from build123d import *

# Parameters (mm, degrees)
SKETCH1_W           = 12.1
SKETCH1_H           = 22.8
BOSS_EXTRUDE1_DEPTH = 24.85
SKETCH2_OUTSIDE_W   = 31.966
SKETCH2_OUTSIDE_H   = 34.016
CUT_EXTRUDE1_DEPTH  = 24.85
SKETCH3_R           = 2.875
SKETCH3_R_2         = 6.05
BOSS_EXTRUDE2_DEPTH = 4.65
BOSS_EXTRUDE3_START = 20.8
BOSS_EXTRUDE3_DEPTH = 2.12
CUT_EXTRUDE2_START  = -2.5
SKETCH6_W           = 12.1
SKETCH6_H           = 22.8
SKETCH6_W_2         = 11.9
SKETCH6_H_2         = 22.6
CUT_EXTRUDE2_DEPTH  = 14
SKETCH8_R           = 3.625
BOSS_EXTRUDE5_DEPTH = 0.3
FILLET1_R           = 0.2
SKETCH9_R           = 2.375
CUT_EXTRUDE3_DEPTH  = 1


with BuildPart() as part:
    # Sketch1 → Boss-Extrude1 (new body)
    with BuildSketch(Plane(origin=(0, 0, 0), x_dir=(1, 0, 0), z_dir=(0, 1, 0))):
        Rectangle(SKETCH1_W, SKETCH1_H)
    extrude(amount=BOSS_EXTRUDE1_DEPTH)

    # Sketch2 outside → Cut-Extrude1 (cut)
    with BuildSketch(Plane.ZY.offset(6.05)):
        with Locations((0, 12.425)):
            Rectangle(SKETCH2_OUTSIDE_W, SKETCH2_OUTSIDE_H)
        Polygon((-11.4, 23.85), (-4.47179677, 24.85), (11.4, 24.85), (11.4, 0), (-11.4, 0), align=None, mode=Mode.SUBTRACT)
    extrude(amount=-CUT_EXTRUDE1_DEPTH, mode=Mode.SUBTRACT)

    # Sketch3 → Boss-Extrude2 (add)
    with BuildSketch(Plane(origin=(0, 24.85, 0), x_dir=(1, 0, 0), z_dir=(0, 1, 0))):
        with Locations((0, 0.325)):
            Circle(SKETCH3_R)
        with Locations((0, -5.35)):
            Circle(SKETCH3_R_2)
        with BuildLine():
            Line((2.875, -0.026760855), (2.875, 0.325))
            ThreePointArc((2.875, 0.325), (2.869926129, 0.154269175), (2.854722425, -0.015859031))
            ThreePointArc((2.854722425, -0.015859031), (2.864866398, -0.021300297), (2.875, -0.026760855))
        make_face()
        with BuildLine():
            ThreePointArc((-2.854722425, -0.015859031), (-2.869926129, 0.154269175), (-2.875, 0.325))
            Line((-2.875, 0.325), (-2.875, -0.026760855))
            ThreePointArc((-2.875, -0.026760855), (-2.864866398, -0.021300297), (-2.854722425, -0.015859031))
        make_face()
    extrude(amount=BOSS_EXTRUDE2_DEPTH)

    # Sketch4 → Boss-Extrude3 (add)
    with BuildSketch(Plane(origin=(0, 0, 0), x_dir=(1, 0, 0), z_dir=(0, 1, 0)).offset(BOSS_EXTRUDE3_START)):
        with BuildLine():
            Line((-6.05, 15.65), (-6.05, 11.4))
            Line((-6.05, 11.4), (6.05, 11.4))
            Line((6.05, 11.4), (6.05, 15.65))
            Line((6.05, 15.65), (0.5, 15.65))
            Line((0.5, 15.65), (0.5, 15.016025404))
            ThreePointArc((0.5, 15.016025404), (0.866025404, 14.65), (1, 14.15))
            ThreePointArc((1, 14.15), (-0.5, 13.283974596), (-0.5, 15.016025404))
            Line((-0.5, 15.016025404), (-0.5, 15.65))
            Line((-0.5, 15.65), (-6.05, 15.65))
        make_face()
        with BuildLine():
            Line((6.05, -11.4), (-6.05, -11.4))
            Line((-6.05, -11.4), (-6.05, -15.65))
            Line((-6.05, -15.65), (-0.5, -15.65))
            Line((-0.5, -15.65), (-0.5, -15.016025404))
            ThreePointArc((-0.5, -15.016025404), (-0.5, -13.283974596), (1, -14.15))
            ThreePointArc((1, -14.15), (0.866025404, -14.65), (0.5, -15.016025404))
            Line((0.5, -15.016025404), (0.5, -15.65))
            Line((0.5, -15.65), (6.05, -15.65))
            Line((6.05, -15.65), (6.05, -11.4))
        make_face()
    extrude(amount=BOSS_EXTRUDE3_DEPTH)

    # Sketch6 → Cut-Extrude2 (cut)
    with BuildSketch(Plane.XZ.offset(CUT_EXTRUDE2_START)):
        Rectangle(SKETCH6_W, SKETCH6_H)
        Rectangle(SKETCH6_W_2, SKETCH6_H_2, mode=Mode.SUBTRACT)
    extrude(amount=-CUT_EXTRUDE2_DEPTH, mode=Mode.SUBTRACT)

    # Sketch8 → Boss-Extrude5 (add)
    with BuildSketch(Plane(origin=(0, 29.5, 0), x_dir=(1, 0, 0), z_dir=(0, 1, 0))):
        with Locations((0, -5.35)):
            Circle(SKETCH8_R)
    extrude(amount=BOSS_EXTRUDE5_DEPTH)

    # Fillet1
    fillet1_edges = [part.edges().sort_by_distance(p)[0] for p in [
        (-3.625, 29.8, 5.35),
    ]]
    fillet(fillet1_edges, radius=FILLET1_R)

    # Sketch9 → Cut-Extrude3 (cut)
    with BuildSketch(Plane(origin=(0, 29.8, 0), x_dir=(1, 0, 0), z_dir=(0, 1, 0))):
        with Locations((0, -5.35)):
            Circle(SKETCH9_R)
    extrude(amount=-CUT_EXTRUDE3_DEPTH, mode=Mode.SUBTRACT)


solid = part.part
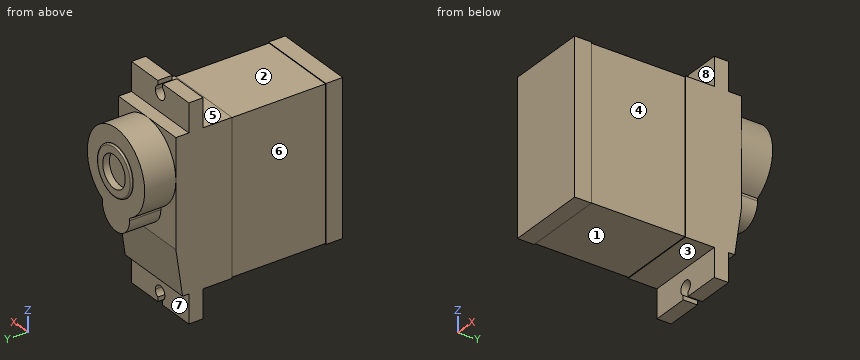
CAD build for the part. Positions are in the model's coordinates, mm. Face numbers are marked on the shaded views. A direction names the side the tool comes from. Coordinates: 2 decimals unless noted, no trailing zeros. Loops run counter-clockwise (first coordinate to the right, second up) from the corner with the lowest first, then second, coordinate; pieces in that order, holes last. Notation, with made-up numbers: (42, 6) - (62, 6) arc R24 ccw to (62, 34) - close; hole circle Ø10 at (52, -0.5). An arc over 180 degrees is marked (long way). Write item = value, one per line. Start each with the question number.
Q1. Drill centre lines: L1, parallel to X at y = 29.1, z = 5.35 (3 decimals); L2, parallel to Z at x = 0, y = 29.55 (3 decimals); L3, parallel to X at y = 3.25, z = -1. Where is each one in solid material? Low to high.
Q2. Cut at D-D, the plane z = -4. List the corners of the cut face in (x, y), then the cut area to 3 significant figures.
Q3. Flat gauge pins, fed straight in: pin 1 Ø5 at (y, z) = (13, 1) entering from +X; pin 2 Ø4 at (y, z) = (8.5, -5) entering from -X; pin 3 Ø1.8 at (x, z) = (0, 14.15) entering from +Y; pin 4 Ø1.3 at (x, z) = (0, 13.5) entering from +Y. Where does each tip first touch, or does it go through?
Q4. Cut at C-C, the plane y = 13.25. List the corners of the cut face in (x, z), then the cut area to 3 significant figures.
Q5. Cut at A-A, the plane z = -8. List the corners of the cut face in (x, y).
Q6. Cut at B-B, the plane x = 4.75. List the corners of the cut face in (y, z).
Q7. Which spindle directions (+Z, -Z, +X, -X, +Y, -Y) get a long thin tool onto all of the face, cutting with end or side? Do the marked faces 1, 2, 3, 4 and 5. Say none if no direction does.
Q8. Pull direction Y, two halves, no side cores. Call the marked faces 6, 7 and 8: pulls with the +Y half, pulls with the -Y half, needs draft (parallel to the pull), parting line crosses it, or undercut.
Computed:
q1.L1 = -6.05 to -2.375, 2.375 to 6.05
q1.L2 = 1.725 to 2.975, 7.725 to 8.975
q1.L3 = -5.95 to 5.95
q2.outline = (-6.05, 0) - (6.05, 0) - (6.05, 2.5) - (5.95, 2.5) - (5.95, 16.5) - (6.05, 16.5) - (6.05, 24.85) - (-6.05, 24.85) - (-6.05, 16.5) - (-5.95, 16.5) - (-5.95, 2.5) - (-6.05, 2.5) - close
q2.area = 298 mm²
q3.pin_1 = 5.95
q3.pin_2 = -5.95
q3.pin_3 = through
q3.pin_4 = 22.92
q4.outline = (-5.95, -11.3) - (5.95, -11.3) - (5.95, 11.3) - (-5.95, 11.3) - close
q4.area = 269 mm²
q5.outline = (-6.05, 0) - (6.05, 0) - (6.05, 2.5) - (5.95, 2.5) - (5.95, 16.5) - (6.05, 16.5) - (6.05, 24.34) - (-6.05, 24.34) - (-6.05, 16.5) - (-5.95, 16.5) - (-5.95, 2.5) - (-6.05, 2.5) - close
q6.outline = (0, -11.4) - (2.5, -11.4) - (2.5, -11.3) - (16.5, -11.3) - (16.5, -11.4) - (20.8, -11.4) - (20.8, -15.65) - (22.92, -15.65) - (22.92, -11.4) - (23.85, -11.4) - (24.85, -4.47) - (24.85, 1.6) - (29.5, 1.6) - (29.5, 9.1) - (24.85, 9.1) - (24.85, 11.4) - (22.92, 11.4) - (22.92, 15.65) - (20.8, 15.65) - (20.8, 11.4) - (16.5, 11.4) - (16.5, 11.3) - (2.5, 11.3) - (2.5, 11.4) - (0, 11.4) - close
q7.face_1 = -Z, +X, -X
q7.face_2 = +Z, +X, -X
q7.face_3 = -Z, +X, -X, -Y
q7.face_4 = +Z, -Z, +X
q7.face_5 = +Z, +X, -X, -Y
q8.face_6 = undercut
q8.face_7 = pulls with the +Y half
q8.face_8 = pulls with the -Y half
